Read the model definition and answer for the solid it produces. Units are mm, in the model's axes. A direction names the side the tool comes from. Coordinates: 2 decimals unless noted, no trailing zeros. Write each loop counter-clockwise with the first axis right and the second up, starting at its lowest first coordinate (ties: lowest second). Pieces come first, ordered by that corner, then holes. Notation, with made-up numbers: (-28, 56) -> (16, 56) arc R13 ccw to (16, 74) -> close; hole circle Ø3 at (82, 56). An arc over 180 degrees is marked (long way). Write item = value, one per line. Start each with the question number.
1) A tool of negligible diameter and unlimited length cuts with its end or side. For faces 5 (the face through (30, -2, -6.35)), 6 (the face through (1.524, -2, -27)), 7 (the face through (-27, -2, -1.524)), 8 (the face through (-26.035, -2, -2)), from which of +Z, -Z, +X, -X, +Y, -Y can it reach the whole face along a straight path? Write none if from no direction.
2) For a pull along Z with two mould halves and no side action, classify faces 1 (the face through (17, -2, -31.75)), 2 (the face through (-27, -2, 1.524)), 3 (the face through (31.75, -2, -4)), 4 (the face through (-18.796, -2, 0)) as released by +Z, released by -Z, zero draft, split by the parting line, or undercut.
3) Section C-C (z = 10.5) is taken. Determine the outline of the cut face in (x, y) (3 decimals), plus the area to 3 significant figures.
4) Section B-B (x = 0) is taken. Determine the outline of the cut face in (y, z) (3 decimals), plus the area to 3 significant figures.
5) Flat-ended cylindrical pins translate along their axes: pin 1 Ø1 at (y, z) = (-2.5, 13) entering from +X (3 decimals); pin 2 Ø1 at (x, y) = (30.5, -2) entering from +Z; pin 3 Ø1 at (y, z) = (-2, 5) entering from -X (3 decimals). Find the tip coordinate at first contact, or state that the pin passes through.
6) Find the intervals of material crossed by line 1 along Z through (x, y) = (3, -1.05) (3 decimals); line 2 along Z through (x, y) = (-26.5, -0.25); line 3 along X through (y, z) = (-0.3, -25.5) (3 decimals), in increasing order. Write a range as from..to.
7) Section A-A (x = -22) is taken. Determine the outline of the cut face in (y, z) (3 decimals).
from build123d import *

# Parameters (mm, degrees)
F0_W     = 63.5
F0_H     = 63.5
F1_DEPTH = 3.175
F2_W     = 3.175
F2_H     = 25.4
F3_DEPTH = 25.4


with BuildPart() as f1:
    # F0 (on Front) → F1 (new body)
    with BuildSketch(Plane.XZ):
        Rectangle(F0_W, F0_H)
    extrude(amount=F1_DEPTH)

    # F2 (on face) → F3 (cut)
    with BuildSketch(Plane.XZ.offset(3.175)):
        with Locations((30.1625, 19.05)):
            Rectangle(F2_W, F2_H)
        with Locations((30.1625, -19.05)):
            Rectangle(F2_W, F2_H)
        Polygon((31.75, 1.905), (27.94, 1.905), (27.94, -1.905), (31.75, -1.905), (31.75, 0), align=None)
        Polygon((-6.35, -31.75), (0, -31.75), (6.35, -31.75), (6.35, -28.575), (1.524, -28.575), (1.524, -26.035), (3.429, -26.035), (3.429, -22.86), (1.524, -22.86), (1.524, -18.796), (0, -18.796), (-1.524, -18.796), (-1.524, -22.86), (-3.429, -22.86), (-3.429, -26.035), (-1.524, -26.035), (-1.524, -28.575), (-6.35, -28.575), align=None)
        Polygon((-31.75, 6.35), (-31.75, 0), (-31.75, -6.35), (-28.575, -6.35), (-28.575, -1.524), (-26.035, -1.524), (-26.035, -3.429), (-22.86, -3.429), (-22.86, -1.524), (-18.796, -1.524), (-18.796, 0), (-18.796, 1.524), (-22.86, 1.524), (-22.86, 3.429), (-26.035, 3.429), (-26.035, 1.524), (-28.575, 1.524), (-28.575, 6.35), align=None)
    extrude(amount=-F3_DEPTH, mode=Mode.SUBTRACT)


solid = f1.part
Answer key:
q1.face_5 = -Z, +X, +Y, -Y
q1.face_6 = -Z, +Y, -Y
q1.face_7 = -X, +Y, -Y
q1.face_8 = +Y, -Y
q2.face_1 = released by -Z
q2.face_2 = undercut
q2.face_3 = zero draft
q2.face_4 = undercut
q3.outline = (-31.75, -3.175) -> (28.575, -3.175) -> (28.575, 0) -> (-31.75, 0) -> close
q3.area = 192 mm^2
q4.outline = (-3.175, -18.796) -> (0, -18.796) -> (0, 31.75) -> (-3.175, 31.75) -> close
q4.area = 160 mm^2
q5.pin_1 = 28.575
q5.pin_2 = 6.35
q5.pin_3 = -28.575
q6.line_1 = -28.575..-26.035, -22.86..31.75
q6.line_2 = -31.75..-1.52, 1.52..31.75
q6.line_3 = -31.75..-3.429, 3.429..28.575
q7.outline = (-3.175, -31.75) -> (0, -31.75) -> (0, -1.524) -> (-3.175, -1.524) -> close; (-3.175, 1.524) -> (0, 1.524) -> (0, 31.75) -> (-3.175, 31.75) -> close
